Source: CAD feature listing. Evaluate the final solid. Frame: model axes, mm. Face numbers are marked on the shaded views. A direction names the side the tool comes from. Coordinates: 2 decimals unless noted, no trailing zeros. Order: outer loops, then holes, each group sorted by start corner. A loop starts at its lowest first (then second) coordinate and runs counter-clockwise, first axis right, second up. Notation, with made-up numbers: (50.25, 34.25) -> (61.25, 34.25) arc R20 ccw to (61.25, 42.25) -> close; hole circle Ø2 at (41.25, 18.5). An arc over 180 degrees is marked (long way). Put each result on its own line as item: value.
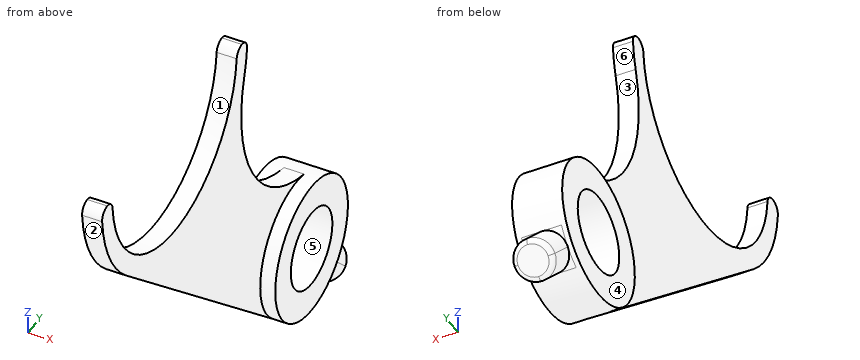
from build123d import *

# Parameters (mm, degrees)
BOSS_EXTRUDE1_DEPTH     = 1
SKETCH1_3_R             = 7
SKETCH1_3_R_2           = 4
BOSS_EXTRUDE2_DEPTH     = 2.5
BOSS_EXTRUDE3_DEPTH     = 2
CUT_EXTRUDE1_REACH      = 61.611
CUT_EXTRUDE1_END_RADIUS = 7
FILLET1_R               = 0.5
FILLET2_START           = -2
FILLET2_DEPTH           = 4
FILLET3_START           = -2
FILLET3_DEPTH           = 4


with BuildPart() as part:
    # Sketch1 → Boss-Extrude1 (new, symmetric)
    with BuildSketch(Plane.YZ):
        with BuildLine():
            Line((-9.247850598, -10.510816301), (18.876074701, -35.255408151))
            ThreePointArc((18.876074701, -35.255408151), (17.246857686, -26.853857727), (24.964224943, -23.154852426))
            ThreePointArc((24.964224943, -23.154852426), (15.014290028, -16.032467293), (13.446719603, -3.896887464))
            ThreePointArc((13.446719603, -3.896887464), (13.860989763, -1.967984445), (14, 0))
            Line((14, 0), (12, 0))
            ThreePointArc((12, 0), (0, -12), (-12, 0))
            Line((-12, 0), (-14, 0))
            ThreePointArc((-14, 0), (-12.756761117, -5.767585788), (-9.247850598, -10.510816301))
        make_face()
    extrude(amount=BOSS_EXTRUDE1_DEPTH, both=True)

    # Sketch1<3> → Boss-Extrude2 (add, symmetric)
    with BuildSketch(Plane.YZ):
        with Locations(Location((23.5, -30, 0), (0, 0, 270))):
            Circle(SKETCH1_3_R)
        with Locations(Location((23.5, -30, 0), (0, 0, 270))):
            Circle(SKETCH1_3_R_2, mode=Mode.SUBTRACT)
    extrude(amount=BOSS_EXTRUDE2_DEPTH, both=True)

    # Sketch1<4> → Boss-Extrude3 (add, symmetric)
    with BuildSketch(Plane.YZ):
        with BuildLine():
            ThreePointArc((29.657630053, -33.329202928), (29.11248608, -34.183300133), (28.449747468, -34.949747468))
            Line((28.449747468, -34.949747468), (31.278174593, -37.778174593))
            Line((31.278174593, -37.778174593), (32.692388155, -36.363961031))
            Line((32.692388155, -36.363961031), (29.657630053, -33.329202928))
        make_face()
        with BuildLine():
            ThreePointArc((28.449747468, -34.949747468), (27.683300133, -35.61248608), (26.829202928, -36.157630053))
            Line((26.829202928, -36.157630053), (29.863961031, -39.192388155))
            Line((29.863961031, -39.192388155), (31.278174593, -37.778174593))
            Line((31.278174593, -37.778174593), (28.449747468, -34.949747468))
        make_face()
    extrude(amount=BOSS_EXTRUDE3_DEPTH, both=True)

    # Cut-Extrude1: up to this cylinder (the profile starts outside it)
    cut_extrude1_end = Plane(origin=(0, 23.5, -30), z_dir=(-1, 0, 0)) * Cylinder(CUT_EXTRUDE1_END_RADIUS, 141.328528, mode=Mode.PRIVATE)
    # Sketch2 → Cut-Extrude1 (cut, up to the surface)
    with BuildSketch(Plane(origin=(0, 34.528174593, -34.528174593), x_dir=(-1, 0, 0), z_dir=(0, 0.707106781186549, -0.7071067811865461)), mode=Mode.PRIVATE) as cut_extrude1_sk1:
        with BuildLine():
            ThreePointArc((-2, -4.596194078), (-1.414213562, -3.181980515), (0, -2.596194078))
            Line((0, -2.596194078), (-2, -2.596194078))
            Line((-2, -2.596194078), (-2, -4.596194078))
        make_face()
    cut_extrude1_tool1 = extrude(cut_extrude1_sk1.sketch, amount=-CUT_EXTRUDE1_REACH, mode=Mode.PRIVATE) - cut_extrude1_end
    add(cut_extrude1_tool1.solids().sort_by_distance((1.553264, 32.376498, -36.679851))[0], mode=Mode.SUBTRACT)
    # Sketch2 → Cut-Extrude1 (cut, up to the surface)
    with BuildSketch(Plane(origin=(0, 34.528174593, -34.528174593), x_dir=(-1, 0, 0), z_dir=(0, 0.707106781186549, -0.7071067811865461)), mode=Mode.PRIVATE) as cut_extrude1_sk2:
        with BuildLine():
            ThreePointArc((0, -2.596194078), (1.414213562, -3.181980515), (2, -4.596194078))
            Line((2, -4.596194078), (2, -2.596194078))
            Line((2, -2.596194078), (0, -2.596194078))
        make_face()
    cut_extrude1_tool2 = extrude(cut_extrude1_sk2.sketch, amount=-CUT_EXTRUDE1_REACH, mode=Mode.PRIVATE) - cut_extrude1_end
    add(cut_extrude1_tool2.solids().sort_by_distance((-1.553264, 32.376498, -36.679851))[0], mode=Mode.SUBTRACT)
    # Sketch2 → Cut-Extrude1 (cut, up to the surface)
    with BuildSketch(Plane(origin=(0, 34.528174593, -34.528174593), x_dir=(-1, 0, 0), z_dir=(0, 0.707106781186549, -0.7071067811865461)), mode=Mode.PRIVATE) as cut_extrude1_sk3:
        with BuildLine():
            Line((1.9e-08, -6.596194078), (2, -6.596194078))
            Line((2, -6.596194078), (2, -4.596194078))
            ThreePointArc((2, -4.596194078), (1.414213569, -6.010407633), (1.9e-08, -6.596194078))
        make_face()
    cut_extrude1_tool3 = extrude(cut_extrude1_sk3.sketch, amount=-CUT_EXTRUDE1_REACH, mode=Mode.PRIVATE) - cut_extrude1_end
    add(cut_extrude1_tool3.solids().sort_by_distance((-1.553264, 30.179851, -38.876498))[0], mode=Mode.SUBTRACT)
    # Sketch2 → Cut-Extrude1 (cut, up to the surface)
    with BuildSketch(Plane(origin=(0, 34.528174593, -34.528174593), x_dir=(-1, 0, 0), z_dir=(0, 0.707106781186549, -0.7071067811865461)), mode=Mode.PRIVATE) as cut_extrude1_sk4:
        with BuildLine():
            Line((-2, -6.596194078), (1.9e-08, -6.596194078))
            ThreePointArc((1.9e-08, -6.596194078), (-1.414213556, -6.010407647), (-2, -4.596194078))
            Line((-2, -4.596194078), (-2, -6.596194078))
        make_face()
    cut_extrude1_tool4 = extrude(cut_extrude1_sk4.sketch, amount=-CUT_EXTRUDE1_REACH, mode=Mode.PRIVATE) - cut_extrude1_end
    add(cut_extrude1_tool4.solids().sort_by_distance((1.553264, 30.179851, -38.876498))[0], mode=Mode.SUBTRACT)

    # Fillet1
    fillet1_edges = [part.edges().sort_by_distance(p)[0] for p in [
        (0, 29.863961031, -39.192388155),
    ]]
    fillet(fillet1_edges, radius=FILLET1_R)

    # Fillet2: read off the stored shape, not the designer's step
    # Fillet2 outline → Fillet2 (cut)
    with BuildSketch(Plane.YZ.offset(FILLET2_START)):
        with BuildLine():
            ThreePointArc((-14, 0), (-13.989625763, -0.538860843), (-13.958518428, -1.076923077))
            add(Edge.make_bspline(
                [(-13.958518428, -1.076923077), (-13.978684128, -0.815545726), (-13.917861816, -0.505978869), (-13.724957355, -0.19992372), (-13.383008233, 5e-09), (-12.961481386, 0)],
                knots=[0, 0, 0, 0, 0, 0, 0.519259304, 0.519259304, 0.519259304, 0.519259304, 0.519259304, 0.519259304], degree=5, weights=[1, 0.792296278, 0.638518602, 0.53866697, 0.492741383, 0.500741842]))
            Line((-12.961481386, 0), (-14, 0))
        make_face()
        with BuildLine():
            Line((-12, 0), (-12.961481386, 0))
            add(Edge.make_bspline(
                [(-12.961481386, 0), (-12.583056271, -4e-09), (-12.270553606, -0.164313436), (-12.073438627, -0.418546888), (-11.982758039, -0.685704598), (-11.964444366, -0.923076923)],
                knots=[0.519259304, 0.519259304, 0.519259304, 0.519259304, 0.519259304, 0.519259304, 1, 1, 1, 1, 1, 1], degree=5, weights=[0.500741842, 0.508148827, 0.561778135, 0.661629767, 0.807703722, 1]))
            ThreePointArc((-11.964444366, -0.923076923), (-11.991107797, -0.461880723), (-12, 0))
        make_face()
    extrude(amount=FILLET2_DEPTH, mode=Mode.SUBTRACT)

    # Fillet3: read off the stored shape, not the designer's step
    # Fillet3 outline → Fillet3 (cut)
    with BuildSketch(Plane.YZ.offset(FILLET3_START)):
        with BuildLine():
            ThreePointArc((12, 0), (11.991107797, -0.461880723), (11.964444366, -0.923076923))
            add(Edge.make_bspline(
                [(11.964444366, -0.923076923), (11.982758039, -0.685704597), (12.073438628, -0.418546886), (12.270553609, -0.164313433), (12.583056275, -2e-09), (12.961481392, 0)],
                knots=[0, 0, 0, 0, 0, 0, 0.480740697, 0.480740697, 0.480740697, 0.480740697, 0.480740697, 0.480740697], degree=5, weights=[1, 0.807703721, 0.661629766, 0.561778134, 0.508148826, 0.500741841]))
            Line((12.961481392, 0), (12, 0))
        make_face()
        with BuildLine():
            Line((14, 0), (12.961481392, 0))
            add(Edge.make_bspline(
                [(12.961481392, 0), (13.383008238, 2e-09), (13.724957357, -0.199923723), (13.917861817, -0.505978871), (13.978684128, -0.815545728), (13.958518427, -1.076923077)],
                knots=[0.480740697, 0.480740697, 0.480740697, 0.480740697, 0.480740697, 0.480740697, 1, 1, 1, 1, 1, 1], degree=5, weights=[0.500741841, 0.492741384, 0.538666971, 0.638518602, 0.792296279, 1]))
            ThreePointArc((13.958518427, -1.076923077), (13.989625763, -0.538860843), (14, 0))
        make_face()
    extrude(amount=FILLET3_DEPTH, mode=Mode.SUBTRACT)


solid = part.part
1. Set-up query: the marked faces 5 and 6. Return all of +Z, -Z, +X, -X, +Y, -Y with unobstructed straight access to the full face (end or side cutting, diameter ignored); none if empty.
Numbers:
face 5: +X, -X
face 6: +X, -X, +Y
2. Cut plane C-C on z = -29. Output: boundary loops of the cut face in (x, y).
Numbers:
outline: (-2.5, 16.57) -> (-1, 16.57) -> (-1, 11.77) -> (1, 11.77) -> (1, 16.57) -> (2.5, 16.57) -> (2.5, 19.63) -> (-2.5, 19.63) -> close; (-2.5, 27.37) -> (2.5, 27.37) -> (2.5, 30.43) -> (-2.5, 30.43) -> close
3. First-contact query: pin 1 (3 mm diameter, centred on x = -2, y = 22.5, fed in from -Z); pin 2 (1.5 mm diameter, centred on x = 0.5, y = -5, fed in from -Z); pin 3 (3 mm diameter, centred on x = -1, y = 8.5, fed in from +Z); pin 4 (6.5 mm diameter, centred on y = 23.5, z = -30, fed in from +X). Flat tips, straight axial feed; report the tip coordinate or a pass-through.
Numbers:
pin 1: stops at z = -37
pin 2: stops at z = -14.91
pin 3: stops at z = -6.63
pin 4: passes through
4. Ray query, line 1 along Y through (x, z) = (-1.05, -30); line 2 along X through (y, z) = (0, -15); line 3 along Z through (x, y) = (-0.1, 24.5). Return the intervals inside material, ascending.
Numbers:
line 1: y = 16.5 to 19.5, 27.5 to 30.5
line 2: x = -1 to 1
line 3: z = -36.93 to -33.87, -26.13 to -23.05
5. Pull-direction query (Y, two-part tool) for the marked faces 1, 2, 3 and 4; classes: pulls with the +Y half, pulls with the -Y half, needs draft (parallel to the pull), parting line crosses it, or undercut.
Numbers:
face 1: undercut
face 2: pulls with the -Y half
face 3: pulls with the +Y half
face 4: needs draft
6. Cut plane B-B on z = -11. Output: boundary loops of the cut face in (x, y).
Numbers:
outline: (-1, -8.69) -> (1, -8.69) -> (1, -4.8) -> (-1, -4.8) -> close; (-1, 4.8) -> (1, 4.8) -> (1, 13.11) -> (-1, 13.11) -> close
7. Cut plane A-A on y = 23.5. Output: boundary loops of the cut face in (x, z).
Numbers:
outline: (-2.5, -37) -> (2.5, -37) -> (2.5, -34) -> (-2.5, -34) -> close; (-2.5, -26) -> (2.5, -26) -> (2.5, -23) -> (1, -23) -> (1, -22.77) -> (-1, -22.77) -> (-1, -23) -> (-2.5, -23) -> close
